Verification items for the finished model (mm, model axes). Face numbers are marked on the shaded views. A direction names the side the tool comes from. Coordinates: 2 decimals unless noted, no trailing zeros. Write each loop counter-clockwise with the first axis right and the second up, starting at its lowest first coordinate (ties: lowest second). Pieces come first, ordered by that corner, then holes. Notation, with made-up numbers: (72.5, -19.75) -> (112.5, -19.75) arc R20 ccw to (112.5, 2.25) -> close; hole circle Ø2 at (20, 9.5). An arc over 180 degrees is marked (long way). Use CSV: the item, a comma, the result in double quotes.
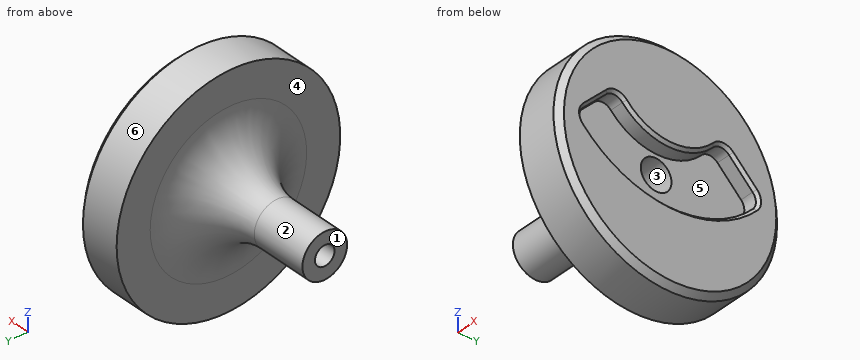
```python
from build123d import *

# Parameters (mm, degrees)
CORTAR_EXTRUIR1_DEPTH = 2.9
REDONDEO1_R           = 10
CORTAR_EXTRUIR2_REACH = 41.799
CROQUIS3_R            = 1.75
CROQUIS4_R            = 2.75
CORTAR_EXTRUIR3_DEPTH = 22.1
CHAFL_N1_SIZE         = 1
CHAFL_N2_SIZE         = 0.5


with BuildPart() as part:
    # Croquis1 → Revolución1 (revolve)
    with BuildSketch(Plane.XY):
        Polygon((-20, 0), (-20, 4), (0, 4), (0, 20), (8, 20), (8, 0), align=None)
    revolve(axis=Axis((8, 0, 0), (-1, 0, 0)))

    # Croquis2 → Cortar-Extruir1 (cut)
    with BuildSketch(Plane(origin=(8, 0, 0), x_dir=(0, 0, -1), z_dir=(1, 0, 0))):
        with BuildLine():
            Line((-2.839199656, 15.194118815), (-7.049029232, 10.984289239))
            ThreePointArc((-7.049029232, 10.984289239), (-7.634375098, 9.528098398), (-6.988431485, 8.097756342))
            ThreePointArc((-6.988431485, 8.097756342), (-3.433318471, 0), (-6.988431485, -8.097756342))
            ThreePointArc((-6.988431485, -8.097756342), (-7.634375098, -9.528098398), (-7.049029232, -10.984289239))
            Line((-7.049029232, -10.984289239), (-2.839199656, -15.194118815))
            ThreePointArc((-2.839199656, -15.194118815), (-1.453779812, -15.779697972), (-0.052075025, -15.234248815))
            ThreePointArc((-0.052075025, -15.234248815), (6.516681529, 0), (-0.052075025, 15.234248815))
            ThreePointArc((-0.052075025, 15.234248815), (-1.453779812, 15.779697972), (-2.839199656, 15.194118815))
        make_face()
    extrude(amount=-CORTAR_EXTRUIR1_DEPTH, mode=Mode.SUBTRACT)

    # Redondeo1
    redondeo1_edges = [part.edges().sort_by_distance(p)[0] for p in [
        (0, -4, 0),
    ]]
    fillet(redondeo1_edges, radius=REDONDEO1_R)

    # Croquis3 → Cortar-Extruir2 (cut, up to next)
    with BuildSketch(Plane.ZY.offset(20), mode=Mode.PRIVATE) as cortar_extruir2_sk1:
        with Locations(Location((0, 0, 0), (0, 0, 270))):
            Circle(CROQUIS3_R)
    cortar_extruir2_tool1 = extrude(cortar_extruir2_sk1.sketch, amount=-CORTAR_EXTRUIR2_REACH, mode=Mode.PRIVATE) & part.part
    add(cortar_extruir2_tool1.solids().sort_by_distance((-20, 0, 0))[0], mode=Mode.SUBTRACT)

    # Croquis4 → Cortar-Extruir3 (cut)
    with BuildSketch(Plane(origin=(5.1, 0, 0), x_dir=(0, 0, -1), z_dir=(1, 0, 0))):
        with Locations(Location((0, 0, 0), (0, 0, 90))):
            Circle(CROQUIS4_R)
    extrude(amount=-CORTAR_EXTRUIR3_DEPTH, mode=Mode.SUBTRACT)

    # Chaflán1
    chafl_n1_edges = [part.edges().sort_by_distance(p)[0] for p in [
        (8, -20, 0),
    ]]
    chamfer(chafl_n1_edges, length=CHAFL_N1_SIZE)

    # Chaflán2
    chafl_n2_edges = [part.edges().sort_by_distance(p)[0] for p in [
        (8, -15.779697972, 1.453779812),
        (8, 0, -6.516681529),
        (8, 15.779697972, 1.453779812),
        (8, 13.089204027, 4.944114444),
        (8, 9.528098398, 7.634375098),
        (8, 0, 3.433318471),
        (8, -9.528098398, 7.634375098),
        (8, -13.089204027, 4.944114444),
    ]]
    chamfer(chafl_n2_edges, length=CHAFL_N2_SIZE)


solid = part.part
```
1) Mould release check, pull along Z, two halves, no side actions. Record for the marked faces 1, 2 and 3: released by +Z, released by -Z, zero draft, split by the parting line, or undercut.
Return value:
face 1,"zero draft"
face 2,"split by the parting line"
face 3,"undercut"
2) Set-up check for the marked faces 4, 5 and 6: record each of +Z, -Z, +X, -X, +Y, -Y from which the full face is reachable in a straight line by a thin tool's end or side.
Return value:
face 4,"-X"
face 5,"+X"
face 6,"+X, -X"
3) Cross-section at A-A (x = 6.25). Record the boundary of the cut face in (y, z).
Return value:
outline,"circle Ø40 at (0, 0); hole (-15.23, 0.05) arc R20.95 ccw to (15.23, 0.05) arc R2 ccw to (15.19, 2.84) -> (10.98, 7.05) arc R2 ccw to (8.1, 6.99) arc R11 cw to (-8.1, 6.99) arc R2 ccw to (-10.98, 7.05) -> (-15.19, 2.84) arc R2 ccw to start"
4) Cross-section at C-C (x = -12.5). Record the boundary of the cut face in (y, z), plus the area to 3 significant figures.
Return value:
outline,"circle Ø8 at (0, 0); hole circle Ø5.5 at (0, 0)"
area,"26.5 mm2"
5) Scan lines: L1, parallel to Z at x = -18.3, y = 0; L2, parallel to X at y = -14, z = 12.5; L3, parallel to Z at x = -11.5, y = 0. Record each from-to range of solid material in increasing order.
Return value:
L1,"-4 to -1.75, 1.75 to 4"
L2,"0 to 8"
L3,"-4 to -2.75, 2.75 to 4"
6) Gauge pin test, flat ends, axial feed: pin 1 (1.5 mm diameter, centred on y = 14, z = 9.5, fed in from -X); pin 2 (2 mm diameter, centred on x = 2.5, z = 15, fed in from -Y); pin 3 (11.5 mm diameter, centred on y = 6, z = 4, fed in from +X); pin 4 (5 mm diameter, centred on x = 1, y = 13, fed in from +Z). Record the tip position at first contact, or that the pin passes through.
Return value:
pin 1,"x = 0"
pin 2,"y = -14.28"
pin 3,"x = 8"
pin 4,"z = 17.02"
7) Cross-section at B-B (y = 0). Record the boundary of the cut face in (x, z), plus the area to 3 significant figures.
Return value:
outline,"(-20, -4) -> (-10, -4) arc R10 cw to (0, -14) -> (0, -20) -> (7, -20) -> (8, -19) -> (8, -7.02) -> (7.5, -6.52) -> (5.1, -6.52) -> (5.1, -2.75) -> (-17, -2.75) -> (-17, -1.75) -> (-20, -1.75) -> close; (-20, 1.75) -> (-17, 1.75) -> (-17, 2.75) -> (5.1, 2.75) -> (5.1, 3.43) -> (7.5, 3.43) -> (8, 3.93) -> (8, 19) -> (7, 20) -> (0, 20) -> (0, 14) arc R10 cw to (-10, 4) -> (-20, 4) -> close"
area,"361 mm2"
